```python
from build123d import *

# Parameters (mm, degrees)
F1_DEPTH = 6.35


with BuildPart() as f1:
    # F0 (on Front) → F1 (new body)
    with BuildSketch(Plane.XZ):
        with BuildLine():
            add(Edge.make_bspline(
                [(0, 29.1454624385), (1.0437938543, 29.092111315), (2.9676615883, 28.9021353997), (3.9769254433, 28.960774908), (4.9135610461, 28.8361106068)],
                knots=[0, 0, 0, 0, 0.5411649205, 1, 1, 1, 1], degree=3))
            add(Edge.make_bspline(
                [(0, 29.1454624385), (-0.9437528923, 29.0972246788), (-2.8725435711, 28.9986389771), (-4.9138774721, 28.7269415704), (-5.9563913383, 28.5881850868)],
                knots=[0, 0, 0, 0, 0.4892977256, 1, 1, 1, 1], degree=3))
            add(Edge.make_bspline(
                [(-5.9563913383, 28.5881850868), (-6.0373155006, 28.0471445059), (-6.2016335657, 26.9485512193), (-6.5093200592, 25.2156363617), (-6.5898328104, 24.0659783815), (-6.62991032, 23.4937034547)],
                knots=[0, 0, 0, 0, 0.3276624402, 0.6653248753, 1, 1, 1, 1], degree=3))
            add(Edge.make_bspline(
                [(-6.62991032, 23.4937034547), (-7.1630712073, 23.3361625005), (-8.2499255604, 23.0150135266), (-9.9572225739, 22.336204538), (-10.8475304186, 21.7288015321), (-11.2771932036, 21.435668692)],
                knots=[0, 0, 0, 0, 0.3325381872, 0.6778827649, 1, 1, 1, 1], degree=3))
            add(Edge.make_bspline(
                [(-11.2771932036, 21.435668692), (-11.8350702765, 21.8249692799), (-13.0377139366, 22.6642041338), (-14.5223554917, 23.7203330679), (-15.3183080256, 24.2865495384)],
                knots=[0, 0, 0, 0, 0.4638756196, 1, 1, 1, 1], degree=3))
            add(Edge.make_bspline(
                [(-15.3183080256, 24.2865495384), (-15.7393330058, 24.0996279574), (-16.6177593429, 23.7096348514), (-17.8974724533, 22.6498262533), (-19.4217291693, 21.176610486), (-20.9120929279, 19.6036415161), (-22.2988027199, 17.9964793951), (-22.7815170567, 17.1662651554), (-22.9964256287, 16.7966466397)],
                knots=[0, 0, 0, 0, 0.1470342518, 0.3067721995, 0.488195784, 0.6741675209, 0.8549365796, 1, 1, 1, 1], degree=3))
            add(Edge.make_bspline(
                [(-22.9964256287, 16.7966466397), (-22.7827786963, 16.4290347992), (-22.3389569602, 15.6653724171), (-21.4374221971, 14.5295552957), (-20.4705705808, 13.2063534042), (-20.054743296, 12.7638344348), (-19.881401211, 12.5793656334)],
                knots=[0, 0, 0, 0, 0.2493452916, 0.5179801039, 0.7990648116, 1, 1, 1, 1], degree=3))
            add(Edge.make_bspline(
                [(-19.881401211, 12.5793656334), (-20.0846392768, 12.2431799217), (-20.5544790803, 11.4659956468), (-21.3840934518, 9.4147652747), (-21.6421566332, 8.1490557932), (-21.7672549188, 7.5354925357)],
                knots=[0, 0, 0, 0, 0.2820132239, 0.6519499051, 1, 1, 1, 1], degree=3))
            add(Edge.make_bspline(
                [(-21.7672549188, 7.5354925357), (-22.4007651503, 7.4617805928), (-23.8174591466, 7.2969414761), (-25.7501887359, 6.9725709243), (-26.8186498433, 6.7932507955)],
                knots=[0, 0, 0, 0, 0.4471750661, 1, 1, 1, 1], degree=3))
            add(Edge.make_bspline(
                [(-26.8186498433, 6.7932507955), (-27.0150206584, 5.7106997675), (-27.4153649769, 3.5036856882), (-27.487576028, -0.1420278505), (-27.1724841229, -2.4576482164), (-26.8158489096, -3.6351135415), (-26.6502574086, -4.1818297468)],
                knots=[0, 0, 0, 0, 0.2787464784, 0.5682848997, 0.7995476925, 1, 1, 1, 1], degree=3))
            add(Edge.make_bspline(
                [(-26.6502574086, -4.1818297468), (-25.6482524067, -4.283882262), (-23.7991424402, -4.4630401598), (-22.4348870789, -4.6582824608), (-21.7444170266, -4.7435350716)],
                knots=[0, 0, 0, 0, 0.5418119861, 1, 1, 1, 1], degree=3))
            add(Edge.make_bspline(
                [(-21.7444170266, -4.7435350716), (-21.5301513936, -5.3239807478), (-20.8973837805, -6.4748096374), (-20.1371624634, -8.4217377612), (-19.7523654924, -9.0446974596), (-19.6018647403, -9.2973606661)],
                knots=[0, 0, 0, 0, 0.3651712445, 0.7411436265, 1, 1, 1, 1], degree=3))
            add(Edge.make_bspline(
                [(-19.6018647403, -9.2973606661), (-19.8557043075, -9.6575667806), (-20.3660684195, -10.5039588883), (-21.8038157451, -12.2702435785), (-22.2412676268, -13.1592855453), (-22.545369342, -13.4900901467)],
                knots=[0, 0, 0, 0, 0.3068371792, 0.6931629329, 1, 1, 1, 1], degree=3))
            add(Edge.make_bspline(
                [(-22.545369342, -13.4900901467), (-22.0940668912, -14.1195692007), (-21.0761124198, -15.5394175013), (-18.599436748, -18.5356038568), (-16.1004309615, -20.144341254), (-15.1952966672, -20.8413432762), (-14.8161659017, -21.133294329)],
                knots=[0, 0, 0, 0, 0.2417916314, 0.5453834162, 0.8095761762, 1, 1, 1, 1], degree=3))
            add(Edge.make_bspline(
                [(-14.8161659017, -21.133294329), (-14.4035545557, -20.8762121849), (-13.5164676765, -20.3235027183), (-11.938800627, -19.0453001605), (-11.1645796897, -18.4402777711), (-10.8113959432, -18.1642789394)],
                knots=[0, 0, 0, 0, 0.321074097, 0.6902878978, 1, 1, 1, 1], degree=3))
            add(Edge.make_bspline(
                [(-10.8113959432, -18.1642789394), (-10.4377997552, -18.356428426), (-9.578418285, -18.7984289431), (-7.4377889326, -19.6846188267), (-6.0846706958, -19.9707083991), (-5.4249824025, -20.1101861894)],
                knots=[0, 0, 0, 0, 0.2826999765, 0.6502933629, 1, 1, 1, 1], degree=3))
            add(Edge.make_bspline(
                [(-5.4249824025, -20.1101861894), (-5.3610155769, -20.6541840451), (-5.2299201103, -21.7690690184), (-4.9868161685, -23.6038968225), (-4.700150649, -24.5945667946), (-4.5639569871, -25.0652302057)],
                knots=[0, 0, 0, 0, 0.3334135521, 0.6833073978, 1, 1, 1, 1], degree=3))
            add(Edge.make_bspline(
                [(-4.5639569871, -25.0652302057), (-4.0036224765, -25.1967327146), (-2.7763592192, -25.4257120062), (-0.8901785241, -25.5282377636), (-0.1930272857, -25.4964662667), (0, -25.538245216)],
                knots=[0, 0, 0, 0, 0.3722930601, 0.7521386883, 1, 1, 1, 1], degree=3))
            add(Edge.make_bspline(
                [(5.9308572672, -24.8031578958), (5.2689139487, -24.9585065411), (2.6790443076, -25.4731548763), (0.9559764293, -25.5156687774), (0.1722671255, -25.5009596091), (0, -25.538245216)],
                knots=[0, 0, 0, 0, 0.4398031871, 0.7787962694, 1, 1, 1, 1], degree=3))
            add(Edge.make_bspline(
                [(6.7557585426, -19.7417400777), (6.688428351, -20.314341258), (6.5813657899, -21.6402709566), (6.2935524423, -23.3259978833), (6.0650862164, -24.3392842162), (5.9308572672, -24.8031578958)],
                knots=[0, 0, 0, 0, 0.350944386, 0.6878759656, 1, 1, 1, 1], degree=3))
            add(Edge.make_bspline(
                [(11.3211954013, -17.6592599601), (10.8213650634, -17.9163346998), (9.7584232665, -18.866459568), (7.3118023933, -19.6875722622), (7.1734705952, -19.6534232853), (6.7557585426, -19.7417400777)],
                knots=[0, 0, 0, 0, 0.3782212702, 0.7785671222, 1, 1, 1, 1], degree=3))
            add(Edge.make_bspline(
                [(15.8065371215, -20.8630748093), (15.3251736992, -20.56315591), (13.8665011648, -19.4558100421), (12.7789681935, -18.8303028026), (11.6959509508, -17.9521162845), (11.3211954013, -17.6592599601)],
                knots=[0, 0, 0, 0, 0.3745736215, 0.6713712616, 1, 1, 1, 1], degree=3))
            add(Edge.make_bspline(
                [(23.0551678687, -13.2540129125), (22.5634664887, -13.9398406075), (21.2969886908, -15.5947202126), (19.3865031013, -17.7631830268), (16.5740495299, -19.9562511424), (16.1467053643, -20.6011269916), (15.8065371215, -20.8630748093)],
                knots=[0, 0, 0, 0, 0.2634359256, 0.5400288837, 0.8291456578, 1, 1, 1, 1], degree=3))
            add(Edge.make_bspline(
                [(19.9714973569, -8.6084809154), (20.2495023641, -9.0029785287), (21.011999566, -10.2999652272), (21.9169868652, -11.70396495), (23.0144243441, -12.8465890354), (23.0551678687, -13.2540129125)],
                knots=[0, 0, 0, 0, 0.3360479736, 0.6730359544, 1, 1, 1, 1], degree=3))
            add(Edge.make_bspline(
                [(21.8937862664, -3.8027581759), (21.7035819832, -4.3180216468), (21.4474562337, -5.4083164729), (20.8218480912, -6.8864413809), (20.1707750268, -8.2739301949), (19.9714973569, -8.6084809154)],
                knots=[0, 0, 0, 0, 0.3241636739, 0.6572489225, 1, 1, 1, 1], degree=3))
            add(Edge.make_bspline(
                [(27.0599387586, -3.2821381465), (26.0380611154, -3.3862146566), (23.9300050389, -3.5368732847), (22.5680630159, -3.7195049586), (21.8937862664, -3.8027581759)],
                knots=[0, 0, 0, 0, 0.5525576762, 1, 1, 1, 1], degree=3))
            add(Edge.make_bspline(
                [(26.8997494131, 7.65088154), (27.1242064519, 6.4134970641), (27.3633651924, 3.5787653193), (27.439365489, -0.1607865373), (27.3473887116, -1.3791971203), (27.2348576602, -2.7046266344), (27.0599387586, -3.2821381465)],
                knots=[0, 0, 0, 0, 0.3186146021, 0.6147483075, 0.7882566602, 1, 1, 1, 1], degree=3))
            add(Edge.make_bspline(
                [(21.693546325, 8.4518361837), (22.3789499151, 8.3720862005), (24.304576792, 8.0593863157), (25.7784109563, 8.0113112926), (26.8997494131, 7.65088154)],
                knots=[0, 0, 0, 0, 0.4838049656, 1, 1, 1, 1], degree=3))
            add(Edge.make_bspline(
                [(19.4108262658, 12.9772247747), (19.6651851258, 12.5564777356), (20.683890471, 11.5867833538), (21.2529723436, 9.3224373945), (21.598601005, 8.9175097099), (21.693546325, 8.4518361837)],
                knots=[0, 0, 0, 0, 0.352948459, 0.7358418825, 1, 1, 1, 1], degree=3))
            add(Edge.make_bspline(
                [(22.6947367191, 17.4225196242), (22.4413821761, 16.9865848375), (21.5126588146, 15.8983840367), (21.1662670639, 15.2110067721), (20.3757160555, 14.255874727), (19.6432982612, 13.2246189971), (19.4108262658, 12.9772247747)],
                knots=[0, 0, 0, 0, 0.2956876643, 0.4893521651, 0.730522428, 1, 1, 1, 1], degree=3))
            add(Edge.make_bspline(
                [(14.6851977333, 25.0315796584), (15.2235059004, 24.7925881059), (16.6051459422, 23.5783271475), (17.8795272181, 22.7063806851), (19.3795101389, 21.1942951621), (20.9703035578, 19.602131019), (21.6083627989, 18.5856925536), (22.4685614557, 17.8115155791), (22.6947367191, 17.4225196242)],
                knots=[0, 0, 0, 0, 0.187992975, 0.3461125439, 0.5256980424, 0.7097856138, 0.8473315558, 1, 1, 1, 1], degree=3))
            add(Edge.make_bspline(
                [(10.480189696, 21.667573601), (11.0545698354, 22.0683904419), (12.4507201039, 23.2125696165), (13.9096179326, 24.4798557319), (14.6851977333, 25.0315796584)],
                knots=[0, 0, 0, 0, 0.4775979441, 1, 1, 1, 1], degree=3))
            add(Edge.make_bspline(
                [(5.7545625605, 23.6699581146), (6.3939497446, 23.4810289011), (8.1266642272, 23.0343498509), (9.3072746554, 22.4757967175), (10.0773108512, 21.9424333843), (10.480189696, 21.667573601)],
                knots=[0, 0, 0, 0, 0.3987926726, 0.6979626253, 1, 1, 1, 1], degree=3))
            add(Edge.make_bspline(
                [(4.9135610461, 28.8361106068), (5.0018057445, 28.2461265834), (5.4317244157, 26.8651315663), (5.3164898818, 25.2755494168), (5.7159192748, 24.2217534645), (5.7545625605, 23.6699581146)],
                knots=[0, 0, 0, 0, 0.3573033365, 0.677301645, 1, 1, 1, 1], degree=3))
        make_face()
        with BuildLine():
            ThreePointArc((-14.3957585096, -7.9261912033), (-17.36002773, -0.2137465224), (-16.3007583469, 7.9805590212))
            Line((-16.3007583469, 7.9805590212), (-14.3957585096, -7.9261912033))
        make_face(mode=Mode.SUBTRACT)
        with BuildLine():
            ThreePointArc((0, -15.6414415687), (-6.3381965817, -14.4787839931), (-11.7763839662, -11.0218161717))
            Line((-11.7763839662, -11.0218161717), (0, -11.0218161717))
            Line((0, -11.0218161717), (11.7763839662, -11.0218161717))
            ThreePointArc((11.7763839662, -11.0218161717), (6.3381965817, -14.4787839931), (0, -15.6414415687))
        make_face(mode=Mode.SUBTRACT)
        with BuildLine():
            Line((14.3957585096, -7.9261912033), (16.3007583469, 7.9805590212))
            ThreePointArc((16.3007583469, 7.9805590212), (17.36002773, -0.2137465224), (14.3957585096, -7.9261912033))
        make_face(mode=Mode.SUBTRACT)
        with BuildLine():
            Line((7.2520091198, 3.2180584967), (0, 16.0014592111))
            Line((0, 16.0014592111), (-7.2520091198, 3.2180584967))
            Line((-7.2520091198, 3.2180584967), (-15.0148840621, 10.4570584372))
            ThreePointArc((-15.0148840621, 10.4570584372), (-8.6577731267, 16.8360140302), (0, 19.3153079599))
            ThreePointArc((0, 19.3153079599), (8.6577731267, 16.8360140302), (15.0148840621, 10.4570584372))
            Line((15.0148840621, 10.4570584372), (7.2520091198, 3.2180584967))
        make_face(mode=Mode.SUBTRACT)
    extrude(amount=F1_DEPTH)


solid = f1.part
```
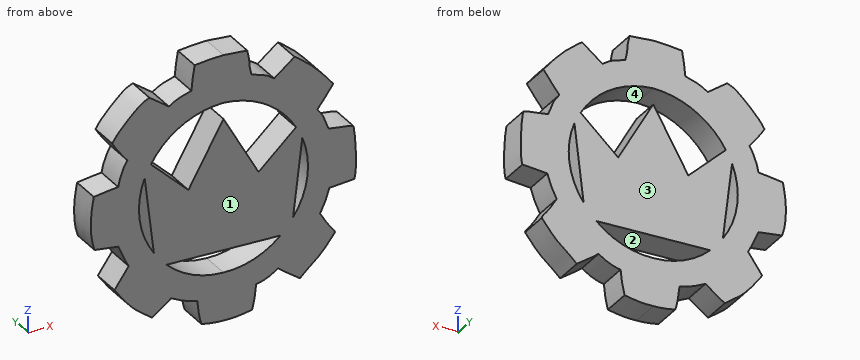
CAD build for the part. Positions are in the model's coordinates, mm. Face numbers are marked on the shaded views. A direction names the side the tool comes from. Round coordinates to 2 decimals unless told otherwise and drop trailing zeros. Answer as CSV lines item,"result". Start each with the question number.
1. Drill centre lines: L1, parallel to Z at x = -20, y = -0.75; L2, parallel to X at y = -1.5, z = -5.5; L3, parallel to Z at x = 7, y = -5.75. Where is each one in solid material? Low to high. Write a range as [from, to].
2. Tool access for the marked faces 3 and 4: list every direction of +Z, -Z, +X, -X, +Y, -Y with a clear straight run to the whole face (end or side of a thin tool).
3. Pin check, flat tips, straight feed: pin 1 (3 mm diameter, centred on y = -4, z = -16, fed in from +X); pin 2 (1.9 mm diameter, centred on x = -3.5, y = -2.5, fed in from -Z); pin 3 (1 mm diameter, centred on y = -4, z = 10, fed in from +X). Stop position of each tip, or through.
4. Saw through at A-A, the plane y = -3.5. Count the separate pieces of the cut face and the enclosed holes in it, and give its area (3 significant figures).
5. Pull direction X, two halves, no side cores. Call the marked faces 1 and 2: +X half, -X half, draft (parallel to the pull), parting line (faces both ways), or undercut.
Model answer:
1,L1,"z = [-16.81, -9.89], [-8.6, 12.38], [12.71, 20.56]"
1,L2,"x = [-21.42, -15.82], [-14.69, 14.69], [15.82, 21.37]"
1,L3,"z = [-19.69, -14.2], [-11.02, 3.66], [17.7, 23.32]"
2,face 3,"+Z, -Z, +X, -X, +Y"
2,face 4,"+Y, -Y"
3,pin 1,"stops at x = 22.13"
3,pin 2,"stops at z = -25.41"
3,pin 3,"stops at x = 21.28"
4,separate pieces,"1"
4,enclosed holes,"4"
4,area,"1,680 mm²"
5,face 1,"draft"
5,face 2,"undercut"
